from build123d import *
from build123d.topology import SkipClean

# Parameters (mm, degrees)
SKETCH1_R           = 14.9
SKETCH1_R_2         = 4
BOSS_EXTRUDE1_DEPTH = 5.5
SKETCH2_R           = 11.5
SKETCH2_R_2         = 4
BOSS_EXTRUDE2_DEPTH = 12
CUT_EXTRUDE2_DEPTH  = 11
CIRPATTERN2_COUNT   = 20
BOSS_EXTRUDE3_START = 1
SKETCH7_R           = 17.5
SKETCH7_R_2         = 4
BOSS_EXTRUDE3_DEPTH = 1
SKETCH8_R           = 17.5
SKETCH8_R_2         = 4
BOSS_EXTRUDE4_DEPTH = 1


with BuildPart() as part:
    # Sketch1 → Boss-Extrude1 (new, symmetric)
    with BuildSketch(Plane(origin=(0, 0, 0), x_dir=(0, 0, -1), z_dir=(1, 0, 0))):
        Circle(SKETCH1_R)
        Circle(SKETCH1_R_2, mode=Mode.SUBTRACT)
    extrude(amount=BOSS_EXTRUDE1_DEPTH, both=True)

    # Sketch2 → Boss-Extrude2 (add)
    with BuildSketch(Plane(origin=(5.5, 0, 0), x_dir=(0, 0, -1), z_dir=(1, 0, 0))):
        Circle(SKETCH2_R)
        Circle(SKETCH2_R_2, mode=Mode.SUBTRACT)
    extrude(amount=BOSS_EXTRUDE2_DEPTH)

    # Sketch6 → Cut-Extrude2 (cut)
    with BuildSketch(Plane.ZY.offset(5.5)):
        Polygon((-1, 12.9), (1, 12.9), (2, 14.9), (-2, 14.9), align=None)
    cut_extrude2 = extrude(amount=-CUT_EXTRUDE2_DEPTH, mode=Mode.SUBTRACT)

    # CirPattern2: Cut-Extrude2 ×20 about axis
    cirpattern2_axis = Axis((0, 0, 0), (1, 0, 0))
    for i in range(1, CIRPATTERN2_COUNT):
        add(cut_extrude2.rotate(cirpattern2_axis, i * 360 / CIRPATTERN2_COUNT), mode=Mode.SUBTRACT)

    # Sketch7 → Boss-Extrude3 (add)
    with SkipClean():  # the faces are left unmerged after this step: merging them gives an invalid solid
        with BuildSketch(Plane.ZY.offset(5.5).offset(BOSS_EXTRUDE3_START)):
            Circle(SKETCH7_R)
            Circle(SKETCH7_R_2, mode=Mode.SUBTRACT)
        extrude(amount=-BOSS_EXTRUDE3_DEPTH)

    # Sketch8 → Boss-Extrude4 (add)
    with SkipClean():  # the faces are left unmerged after this step: merging them gives an invalid solid
        with BuildSketch(Plane(origin=(5.5, 0, 0), x_dir=(0, 0, -1), z_dir=(1, 0, 0))):
            with Locations(Location((0, 0, 0), (0, 0, 180))):
                Circle(SKETCH8_R)
            with Locations(Location((0, 0, 0), (0, 0, 180))):
                Circle(SKETCH8_R_2, mode=Mode.SUBTRACT)
        extrude(amount=BOSS_EXTRUDE4_DEPTH)
    add(part.part.scale(1), mode=Mode.REPLACE)  # the faces are merged on a copy


solid = part.part
Geometry: final body of the model. Coordinates: model frame, mm. A direction names the side the tool comes from. Round coordinates to 2 decimals unless told otherwise and drop trailing zeros. Order: outer loops, then holes, each group sorted by start corner. A loop starts at its lowest first (then second) coordinate and runs counter-clockwise, first axis right, second up. Notation, with made-up numbers: (-8, 15.5) -> (31, 15.5) arc R13 ccw to (31, 22.5) -> close; hole circle Ø5 at (87.25, 75.25). An arc over 180 degrees is marked (long way). Put each result on its own line as item: value. Start each with the question number.
Q1. Pull-direction query (Y, two-part tool) for faces 4 (the flat face through (-6.5, -4, 4)), 5 (the flat face through (-0.08, 2.88, 13.6)), 6 (the flat face through (-0.077, 12.716, -5.683)); classes: +Y half, -Y half, draft (parallel to the pull), parting line (faces both ways), or undercut.
Q2. Section A-A on z = 0. Return the cut outline in (x, y).
Q3. Section C-C on x = 8.75. Return the cut outline in (y, z), and give its area (3 significant figures).
Q4. Reachability of faces 1 (the flat face through (-0.077, 6.948, -12.072)), 2 (the flat face through (-0.077, -12.072, -6.948)), 3 (the flat face through (-0.08, 7.59, 10.43)) from +Z, -Z, +X, -X, +Y, -Y: full face, straight path, thin tool, end or side. Return the list, or none.
Q5. Section B-B on z = -14. Return the cut outline in (x, y), and give its area (3 significant figures).
Q6. First-contact query: pin 1 (3 mm diameter, centred on x = 2, z = 8.5, fed in from -Y); pin 2 (2 mm diameter, centred on x = -3.5, y = 10, fed in from -Z); pin 3 (1 mm diameter, centred on x = -2, y = 0, fed in from -Z). Flat tips, straight axial feed; report the tip coordinate or a pass-through.
Q7. Line query: probe 1 along X at (y, z) = (-7, -14); probe 2 along Z at (x, y) = (-1.5, 0); probe 3 along Y at (x, z) = (-6.2, 0). Output: solid intervals per line, ascending.
Ans:
1. face 4: draft
1. face 5: undercut
1. face 6: +Y half
2. outline: (-6.5, -17.5) -> (-5.5, -17.5) -> (-5.5, -12.9) -> (5.5, -12.9) -> (5.5, -17.5) -> (6.5, -17.5) -> (6.5, -11.5) -> (17.5, -11.5) -> (17.5, -4) -> (-6.5, -4) -> close; (-6.5, 4) -> (17.5, 4) -> (17.5, 11.5) -> (6.5, 11.5) -> (6.5, 17.5) -> (5.5, 17.5) -> (5.5, 12.9) -> (-5.5, 12.9) -> (-5.5, 17.5) -> (-6.5, 17.5) -> close
3. outline: circle Ø23 at (0, 0); hole circle Ø8 at (0, 0)
3. area: 365 mm2
4. face 1: +Y
4. face 2: -Z
4. face 3: none
5. outline: (-6.5, -10.5) -> (-5.5, -10.5) -> (-5.5, -2.82) -> (5.5, -2.82) -> (5.5, -10.5) -> (6.5, -10.5) -> (6.5, 10.5) -> (5.5, 10.5) -> (5.5, 2.82) -> (-5.5, 2.82) -> (-5.5, 10.5) -> (-6.5, 10.5) -> close; hole (-5.5, -1.55) -> (5.5, -1.55) -> (5.5, 1.55) -> (-5.5, 1.55) -> close
5. area: 70.0 mm2
6. pin 1: stops at y = -13.15
6. pin 2: stops at z = -10.81
6. pin 3: stops at z = -12.9
7. probe 1: x = -6.5 to -5.5, 5.5 to 6.5
7. probe 2: z = -12.9 to -4, 4 to 12.9
7. probe 3: y = -17.5 to -4, 4 to 17.5
